from build123d import *

# Parameters (mm, degrees)
SKETCH1_W               = 60
SKETCH1_H               = 50
SKETCH1_W_2             = 55
SKETCH1_H_2             = 45
BOSS_EXTRUDE1_DEPTH     = 50
SKETCH2_W               = 60
SKETCH2_H               = 50
BOSS_EXTRUDE2_DEPTH     = 5
CUT_EXTRUDE1_REACH      = 87.147
SKETCH3_W               = 20
SKETCH3_H               = 5
SKETCH4_W               = 25.74299971
SKETCH4_H               = 5.966870814
BOSS_EXTRUDE5_DEPTH     = 10
SKETCH8_W               = 93.117720322
SKETCH8_H               = 6.00994507
BOSS_EXTRUDE6_DEPTH     = 5
SKETCH10_W              = 60
SKETCH10_H              = 50
SKETCH10_W_2            = 55
SKETCH10_H_2            = 45
BOSS_EXTRUDE7_DEPTH     = 10
CUT_EXTRUDE2_DEPTH      = 123.723278076
CUT_EXTRUDE2_DEPTH_BACK = 123.723278076
SKETCH11_W              = 45
SKETCH11_H              = 3.5


with BuildPart() as part:
    # Sketch1 → Boss-Extrude1 (new body)
    with BuildSketch(Plane(origin=(0, 0, 0), x_dir=(1, 0, 0), z_dir=(0, 1, 0))):
        Rectangle(SKETCH1_W, SKETCH1_H)
        Rectangle(SKETCH1_W_2, SKETCH1_H_2, mode=Mode.SUBTRACT)
    extrude(amount=BOSS_EXTRUDE1_DEPTH)

    # Sketch2 → Boss-Extrude2 (add)
    with BuildSketch(Plane(origin=(0, 50, 0), x_dir=(1, 0, 0), z_dir=(0, 1, 0))):
        Rectangle(SKETCH2_W, SKETCH2_H)
    extrude(amount=BOSS_EXTRUDE2_DEPTH)

    # Sketch3 → Cut-Extrude1 (cut, up to next)
    with BuildSketch(Plane(origin=(30, 0, 0), x_dir=(0, 0, -1), z_dir=(1, 0, 0)), mode=Mode.PRIVATE) as cut_extrude1_sk1:
        with Locations((0, 29.65624639)):
            Rectangle(SKETCH3_W, SKETCH3_H)
    cut_extrude1_tool1 = extrude(cut_extrude1_sk1.sketch, amount=-CUT_EXTRUDE1_REACH, mode=Mode.PRIVATE) & part.part
    add(cut_extrude1_tool1.solids().sort_by_distance((30, 29.656246, 0))[0], mode=Mode.SUBTRACT)

    # Sketch4 → Boss-Extrude5 (add)
    with BuildSketch(Plane(origin=(0, 55, 0), x_dir=(1, 0, 0), z_dir=(0, 1, 0))):
        with Locations((-21.74634114, 0)):
            Rectangle(SKETCH4_W, SKETCH4_H)
    extrude(amount=BOSS_EXTRUDE5_DEPTH)

    # Sketch8 → Boss-Extrude6 (add)
    with BuildSketch(Plane(origin=(0, 65, 0), x_dir=(1, 0, 0), z_dir=(0, 1, 0))):
        with Locations((24.490647417, -0.021537128)):
            Rectangle(SKETCH8_W, SKETCH8_H)
    extrude(amount=-BOSS_EXTRUDE6_DEPTH)

    # Sketch10 → Boss-Extrude7 (add)
    with BuildSketch(Plane.XZ):
        Rectangle(SKETCH10_W, SKETCH10_H)
        Rectangle(SKETCH10_W_2, SKETCH10_H_2, mode=Mode.SUBTRACT)
    extrude(amount=BOSS_EXTRUDE7_DEPTH)

    # Sketch11 → Cut-Extrude2 (cut, two sides: drawn at the far end of the back side and taken through both)
    with BuildSketch(Plane.ZY.offset(30).offset(-CUT_EXTRUDE2_DEPTH_BACK)):
        with Locations((0.11957715, -4.695440094)):
            Rectangle(SKETCH11_W, SKETCH11_H)
    extrude(amount=CUT_EXTRUDE2_DEPTH + CUT_EXTRUDE2_DEPTH_BACK, mode=Mode.SUBTRACT)


solid = part.part
Verification items for the finished model (mm, model axes). A direction names the side the tool comes from. Give positions to 0.01 mm unless a question says otherwise; leave off trailing zeros. Order: outer loops, then holes, each group sorted by start corner. A loop starts at its lowest first (then second) coordinate and runs counter-clockwise, first axis right, second up. Notation, with made-up numbers: M 3.25,17.5 L 36.25,17.5 A20 ccw 36.25,22.5 Z; hole C 35.5,-30 d10. An arc over 180 degrees is marked long. Answer as a JSON object with one key per item and string values. Group by question number.
1) Cross-section at D-D (z = 12). Enter the section's corners in (x, y), then the cut area to 4 significant figures.
2) Cross-section at B-B (z = 0.5). Enter the section's corners in (x, y).
3) Scan lines: line 1 along X through (y, z) = (9.5, 7); line 2 along Z through (x, y) = (12, 38); line 3 along Z through (x, y) = (-15.5, 57.5). Record each from-to range of solid material in increasing order. Write a range as [from, to].
4) Access from +Z, -Z, +X, -X, +Y, -Y to the whole of each face (thin tool, end or side, straight path). Record for faces 4 (the face through (0, 24, 22.5)), 5 (the face through (29, -6.445, 0)), 6 (the face through (29, 30, -10)).
5) Cross-section at C-C (y = 14). Enter the section's corners in (x, z).
6) Cross-section at A-A (x = 23.5). Enter the section's corners in (y, z), then the cut area to 3 significant figures.
7) Mould release check, pull along Z, two halves, no side actions. Record for faces 1 (the face through (-34.618, 60, 0)), 2 (the face through (0, -5, 22.62)), 3 (the face through (24, 63, 3.027)): released by +Z, released by -Z, zero draft, split by the parting line, or undercut.
8) Depth check by flat-ended pin: pin 1 Ø1.5 at (x, z) = (46.5, -3.5) entering from -Y; pin 2 Ø2.5 at (x, y) = (19.5, 63) entering from +Z; pin 3 Ø1.8 at (x, z) = (15, -1.5) entering from -Y. Enter the tip coordinate at first touch or a pass-through.
Result sheet:
{
 "1": {"outline": "M -30,-10 L -27.5,-10 L -27.5,-6.45 L -30,-6.45 Z; M -30,-2.95 L -27.5,-2.95 L -27.5,50 L 27.5,50 L 27.5,-2.95 L 30,-2.95 L 30,55 L -30,55 Z; M 27.5,-10 L 30,-10 L 30,-6.45 L 27.5,-6.45 Z", "area": "582.5 mm2"},
 "2": {"outline": "M -34.62,55 L -30,55 L -30,-2.95 L -27.5,-2.95 L -27.5,50 L 27.5,50 L 27.5,32.16 L 30,32.16 L 30,55 L -8.87,55 L -8.87,60 L 71.05,60 L 71.05,65 L -34.62,65 Z; M -30,-10 L -27.5,-10 L -27.5,-6.45 L -30,-6.45 Z; M 27.5,-10 L 30,-10 L 30,-6.45 L 27.5,-6.45 Z; M 27.5,-2.95 L 30,-2.95 L 30,27.16 L 27.5,27.16 Z"},
 "3": {"line 1": "x = [-30, -27.5], [27.5, 30]", "line 2": "z = [-25, -22.5], [22.5, 25]", "line 3": "z = [-2.98, 2.98]"},
 "4": {"face 4": "-Y", "face 5": "+X, -X", "face 6": "+X"},
 "5": {"outline": "M -30,-25 L 30,-25 L 30,25 L -30,25 Z; hole M -27.5,-22.5 L 27.5,-22.5 L 27.5,22.5 L -27.5,22.5 Z"},
 "6": {"outline": "M -10,-25 L 55,-25 L 55,25 L -10,25 L -10,22.5 L -6.45,22.5 L -6.45,22.62 L -2.95,22.62 L -2.95,22.5 L 50,22.5 L 50,-22.5 L -10,-22.5 Z; M 60,-2.98 L 65,-2.98 L 65,3.03 L 60,3.03 Z", "area": "580 mm2"},
 "7": {"face 1": "zero draft", "face 2": "undercut", "face 3": "released by +Z"},
 "8": {"pin 1": "stops at y = 60", "pin 2": "stops at z = 3.03", "pin 3": "stops at y = 50"}
}
